Answer from the drawing. Dimensions are ordinates in mm from the lowest x, y and z of the part. Coordinates: 2 decimals unless noted, no trailing zeros. Write each loop counter-clockwise with the first axis right and the second up, starting at its lowest first coordinate (ties: lowest second). Pieces come first, ordered by that corner, then holes. Notation, with made-up numbers: (79.5, 82.25) -> (86.5, 82.25) arc R15 cw to (86.5, 101.25) -> close; hole circle Ø6 at (36, -36.5). An arc over 180 degrees is marked (long way). One line per item, written item: value. Start each with the question number.
1. Consider line 1 along Z through (x, y) = (10.25, 43); line 2 along X through (y, z) = (7.5, 4.25); line 3 along Z through (x, y) = (4.5, 8.5). Determine where each line is inside the solid, lowest interval first.
2. Find section A-A, the plane x = 7.75. Write down the section's boundary in (y, z), and give its area (3 significant figures).
3. Find section C-C, the plane y = 43. Write down the section's boundary in (x, z), and give its area (3 significant figures).
4. Find section D-D, the plane x = 10.5. Write down the section's boundary in (y, z).
5. Find section B-B, the plane z = 1.5. Write down the section's boundary in (x, y).
6. For a pull along Y with two mould halves and no side action, classify the marked faces 1, 2 and 3 as pulls with the +Y half, pulls with the -Y half, needs draft (parallel to the pull), parting line crosses it, or undercut.
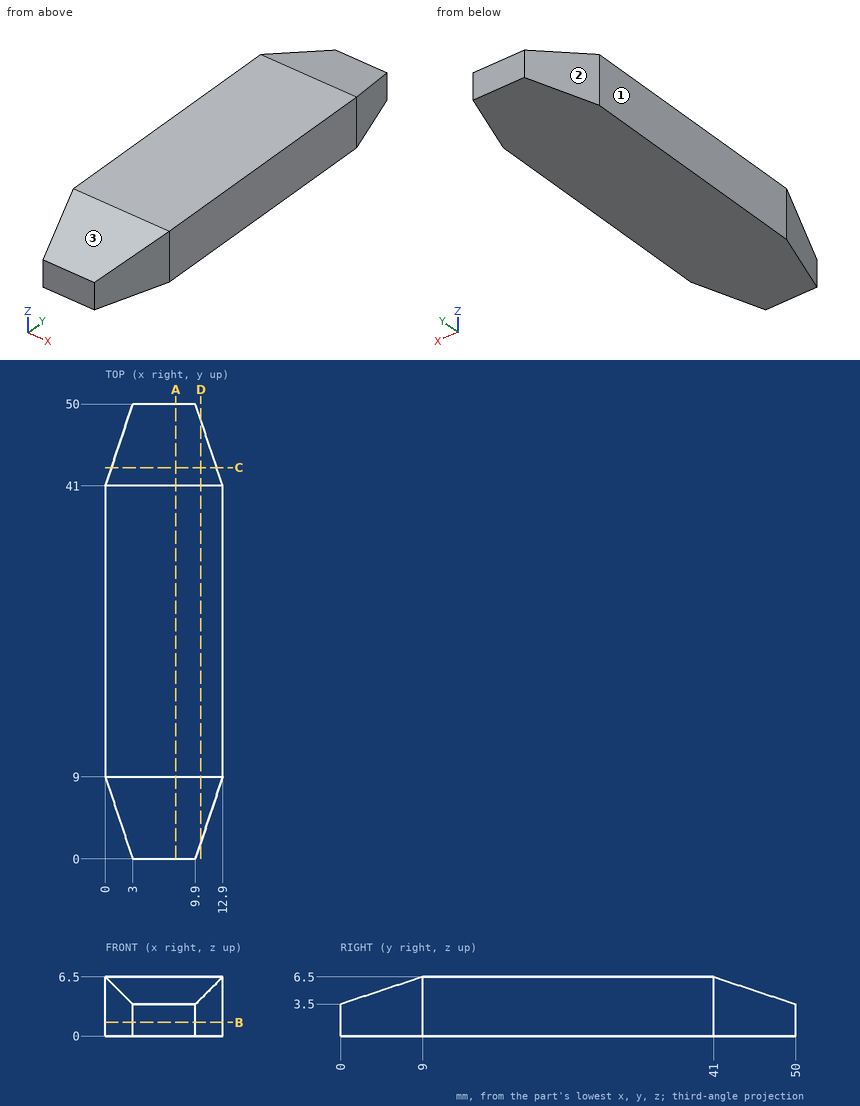
Answer block:
1. line 1: z = 0 to 5.83
1. line 2: x = 0.5 to 12.4
1. line 3: z = 0 to 6.33
2. outline: (0, 0) -> (50, 0) -> (50, 3.5) -> (41, 6.5) -> (9, 6.5) -> (0, 3.5) -> close
2. area: 298 mm2
3. outline: (0.67, 0) -> (12.23, 0) -> (12.23, 5.83) -> (0.67, 5.83) -> close
3. area: 67.5 mm2
4. outline: (1.8, 0) -> (48.2, 0) -> (48.2, 4.1) -> (41, 6.5) -> (9, 6.5) -> (1.8, 4.1) -> close
5. outline: (0, 9) -> (3, 0) -> (9.9, 0) -> (12.9, 9) -> (12.9, 41) -> (9.9, 50) -> (3, 50) -> (0, 41) -> close
6. face 1: needs draft
6. face 2: pulls with the +Y half
6. face 3: pulls with the -Y half
